from build123d import *

# Parameters (mm, degrees)
SKETCH1_W           = 25.4
SKETCH1_H           = 25.4
SKETCH1_W_2         = 19.05
SKETCH1_H_2         = 19.05
BOSS_EXTRUDE1_DEPTH = 164.8
SKETCH2_W           = 22.225
SKETCH2_H           = 25.4
CUT_EXTRUDE1_DEPTH  = 50.8
SKETCH3_W           = 22.225
SKETCH3_H           = 25.4
CUT_EXTRUDE2_DEPTH  = 50.8
SKETCH4_R           = 1.4732
CUT_EXTRUDE3_DEPTH  = 50.8


with BuildPart() as part:
    # Sketch1 → Boss-Extrude1 (new body)
    with BuildSketch(Plane(origin=(0, 0, 0), x_dir=(0, 0, -1), z_dir=(1, 0, 0))):
        with Locations((3.400546448, -4.580327869)):
            Rectangle(SKETCH1_W, SKETCH1_H)
        with Locations((3.400546448, -4.580327869)):
            Rectangle(SKETCH1_W_2, SKETCH1_H_2, mode=Mode.SUBTRACT)
    extrude(amount=BOSS_EXTRUDE1_DEPTH)

    # Sketch2 → Cut-Extrude1 (cut)
    with BuildSketch(Plane(origin=(164.8, 0, 0), x_dir=(0, 0, -1), z_dir=(1, 0, 0))):
        with Locations((4.988046448, -4.580327869)):
            Rectangle(SKETCH2_W, SKETCH2_H)
    extrude(amount=-CUT_EXTRUDE1_DEPTH, mode=Mode.SUBTRACT)

    # Sketch3 → Cut-Extrude2 (cut)
    with BuildSketch(Plane.ZY):
        with Locations((-4.988046448, -4.580327869)):
            Rectangle(SKETCH3_W, SKETCH3_H)
    extrude(amount=-CUT_EXTRUDE2_DEPTH, mode=Mode.SUBTRACT)

    # Sketch4 → Cut-Extrude3 (cut)
    with BuildSketch(Plane.XY.offset(9.299453552)):
        with Locations((19.05, 1.769672131)):
            Circle(SKETCH4_R)
        with Locations(Location((31.75, 1.769672131, 0), (0, 0, 180))):
            Circle(SKETCH4_R)
        with Locations((31.75, -10.930327869)):
            Circle(SKETCH4_R)
        with Locations(Location((19.05, -10.930327869, 0), (0, 0, 180))):
            Circle(SKETCH4_R)
        with Locations((145.75, -10.930327869)):
            Circle(SKETCH4_R)
        with Locations(Location((133.05, -10.930327869, 0), (0, 0, 180))):
            Circle(SKETCH4_R)
        with Locations((133.05, 1.769672131)):
            Circle(SKETCH4_R)
        with Locations(Location((145.75, 1.769672131, 0), (0, 0, 180))):
            Circle(SKETCH4_R)
    extrude(amount=-CUT_EXTRUDE3_DEPTH, mode=Mode.SUBTRACT)


solid = part.part
Source: CAD feature listing. Evaluate the final solid. Frame: model axes, mm. A direction names the side the tool comes from. Coordinates: 2 decimals unless noted, no trailing zeros. Loops run counter-clockwise (first coordinate to the right, second up) from the corner with the lowest first, then second, coordinate; pieces in that order, holes last. Notation, with made-up numbers: (89.25, 0) -> (104.25, 0) arc R26 cw to (104.25, 19) -> close; hole circle Ø4 at (-2, 21). An arc over 180 degrees is marked (long way). Answer in a Markdown table with one row per item. Add a question column.
Q1. Section C-C on y = -4. Return the cut outline in (x, z).
Q2. Section A-A on z = 1.5. Return the cut outline in (x, y).
Q3. Reachability of faces 5 (the face through (81, 8.12, 0)), 6 (the face through (114, -4.5, -13.2)), 7 (the face through (82, -5, -12.926)) from +Z, -Z, +X, -X, +Y, -Y: full face, straight path, thin tool, end or side. Return the list, or none.
Q4. Pull-direction query (Z, two-part tool) for faces 1 (the face through (81, -5, 9.299)), 2 (the face through (82, 4.945, -3)), 3 (the face through (50.8, -5.5, -13.3)), 4 (the face through (82, -5, -16.101)); classes: pulls with the +Z half, pulls with the -Z half, needs draft (parallel to the pull), parting line crosses it, or undercut.
Q5. Contact query for a flat-ended pin moving along its axis: pin 1 Ø12 at (y, z) = (-9.5, -5) entering from +X. Output: stop coordinate, or through.
Q6. Ray query, line 1 along Y through (x, z) = (31.75, 7.3); line 2 along Y through (x, z) = (96.5, -12.5); line 3 along X through (y, z) = (-2.75, -14.5). Return the intervals inside material, ascending.
Q7. Section B-B on x = 145.75. Return the cut outline in (y, z).
Q8. Section D-D on x = 45. Return the cut outline in (y, z), and give its area (3 significant figures).
Computed values:
| question | item | result |
|---|---|---|
| 1 | outline | (0, 6.12) -> (164.8, 6.12) -> (164.8, 9.3) -> (0, 9.3) -> close; (50.8, -16.1) -> (114, -16.1) -> (114, -12.93) -> (50.8, -12.93) -> close |
| 2 | outline | (50.8, -17.28) -> (114, -17.28) -> (114, -14.11) -> (50.8, -14.11) -> close; (50.8, 4.94) -> (114, 4.94) -> (114, 8.12) -> (50.8, 8.12) -> close |
| 3 | face 5 | +Z, -Z, +X, -X, +Y |
| 3 | face 6 | -Z, +X, +Y, -Y |
| 3 | face 7 | +X, -X |
| 4 | face 1 | pulls with the +Z half |
| 4 | face 2 | undercut |
| 4 | face 3 | needs draft |
| 4 | face 4 | pulls with the -Z half |
| 5 | pin 1 | stops at x = 114 |
| 6 | line 1 | y = -17.28 to -12.4, -9.46 to 0.3, 3.24 to 8.12 |
| 6 | line 2 | y = -17.28 to -14.11, 4.94 to 8.12 |
| 6 | line 3 | x = 50.8 to 114 |
| 7 | outline | (-17.28, 6.12) -> (-12.4, 6.12) -> (-12.4, 9.3) -> (-17.28, 9.3) -> close; (-9.46, 6.12) -> (0.3, 6.12) -> (0.3, 9.3) -> (-9.46, 9.3) -> close; (3.24, 6.12) -> (8.12, 6.12) -> (8.12, 9.3) -> (3.24, 9.3) -> close |
| 8 | outline | (-17.28, 6.12) -> (8.12, 6.12) -> (8.12, 9.3) -> (-17.28, 9.3) -> close |
| 8 | area | 80.6 mm^2 |
